```python
from build123d import *

# Parameters (mm, degrees)
SKETCH1_R           = 57.15
BOSS_EXTRUDE1_DEPTH = 2.54
SKETCH3_W           = 55.958888442
SKETCH3_H           = 22.106904705
CUT_EXTRUDE1_DEPTH  = 2.54
SKETCH4_R           = 12.7
CUT_EXTRUDE2_DEPTH  = 2.54
SKETCH5_R           = 12.7
CUT_EXTRUDE3_DEPTH  = 2.54


with BuildPart() as part:
    # Sketch1 → Boss-Extrude1 (new body)
    with BuildSketch(Plane(origin=(0, 0, 0), x_dir=(1, 0, 0), z_dir=(0, 1, 0))):
        Circle(SKETCH1_R)
    extrude(amount=BOSS_EXTRUDE1_DEPTH)

    # Sketch3 → Cut-Extrude1 (cut)
    with BuildSketch(Plane(origin=(0, 2.54, 0), x_dir=(1, 0, 0), z_dir=(0, 1, 0))):
        with Locations((-10.970545038, 0.068604303)):
            Rectangle(SKETCH3_W, SKETCH3_H)
    extrude(amount=-CUT_EXTRUDE1_DEPTH, mode=Mode.SUBTRACT)

    # Sketch4 → Cut-Extrude2 (cut)
    with BuildSketch(Plane(origin=(0, 0, 0), x_dir=(-1, 0, 0), z_dir=(0, -1, 0))):
        with Locations((50.8, 0)):
            Circle(SKETCH4_R)
    extrude(amount=-CUT_EXTRUDE2_DEPTH, mode=Mode.SUBTRACT)

    # Sketch5 → Cut-Extrude3 (cut)
    with BuildSketch(Plane.XZ):
        with Locations((50.8, 0)):
            Circle(SKETCH5_R)
    extrude(amount=-CUT_EXTRUDE3_DEPTH, mode=Mode.SUBTRACT)


solid = part.part
```
Source: CAD feature listing. Evaluate the final solid. Frame: model axes, mm. A direction names the side the tool comes from. Round coordinates to 2 decimals unless told otherwise and drop trailing zeros. Loops run counter-clockwise (first coordinate to the right, second up) from the corner with the lowest first, then second, coordinate; pieces in that order, holes last. Notation, with made-up numbers: M -9,-22 L 9,-22 A36 cw 9,15 Z; hole C 28.25,72 d9. An arc over 180 degrees is marked long. Use a Markdown table: item, result. Add a question column.
1. Pull-direction query (X, two-part tool) for faces 3 (the flat face through (-1, 2.54, 12)), 4 (the flat face through (17.009, 1, 0)), 5 (the cylindrical face through (-1.09, 1.25, 57.14)); classes: +X half, -X half, draft (parallel to the pull), parting line (faces both ways), or undercut.
2. Contact query for flat-ended pins moving along their axis: pin 1 (12 mm diameter, centred on x = 21.5, z = 9.5, fed in from -Y); pin 2 (1.5 mm diameter, centred on x = -43, y = 2, fed in from -Z); pin 3 (1.3 mm diameter, centred on y = 1, z = 7.5, fed in from +X); pin 4 (0.8 mm diameter, centred on y = 1.5, z = 2.5, fed in from -X). Output: stop coordinate, or through.
3. Cut plane A-A, the plane x = 50.8. Output: boundary loops of the cut face in (y, z), and give its area (3 significant figures).
4. Cut plane B-B, the plane y = 0.8. Output: boundary loops of the cut face in (x, z).
5. Cut plane C-C, the plane x = -23. Output: boundary loops of the cut face in (y, z).
6. Ray query, line 1 along X through (y, z) = (0.55, 0); line 2 along Z through (x, y) = (5, 1.55); line 3 along Z through (x, y) = (1, 1.95). Return the intervals inside material, ascending. Write a range as [from, to].
7. Set-up query: faces 1 (the flat face through (-1, 0, 12)), 2 (the flat face through (-38.95, 1, 8)). Return all of +Z, -Z, +X, -X, +Y, -Y with unobstructed straight access to the full face (end or side cutting, diameter ignored); none if empty.
8. Cut plane D-D, the plane z = 0. Output: boundary loops of the cut face in (x, y).
Solution:
| question | item | result |
|---|---|---|
| 1 | face 3 | draft |
| 1 | face 4 | undercut |
| 1 | face 5 | parting line |
| 2 | pin 1 | stops at y = 0 |
| 2 | pin 2 | stops at z = -38.48 |
| 2 | pin 3 | stops at x = 41.06 |
| 2 | pin 4 | stops at x = 17.01 |
| 3 | outline | M 0,-26.18 L 2.54,-26.18 L 2.54,-12.7 L 0,-12.7 Z; M 0,12.7 L 2.54,12.7 L 2.54,26.18 L 0,26.18 Z |
| 3 | area | 68.5 mm2 |
| 4 | outline | M -55.96,-11.6 A57.15 ccw 55.96,-11.6 A12.7 cw long 55.96,11.6 A57.15 ccw -55.96,11.6 A12.7 cw -38.95,4.57 L -38.95,10.98 L 17.01,10.98 L 17.01,-11.12 L -38.95,-11.12 L -38.95,-4.57 A12.7 cw Z |
| 5 | outline | M 0,-52.32 L 2.54,-52.32 L 2.54,-11.12 L 0,-11.12 Z; M 0,10.98 L 2.54,10.98 L 2.54,52.32 L 0,52.32 Z |
| 6 | line 1 | x = [17.01, 38.1] |
| 6 | line 2 | z = [-56.93, -11.12], [10.98, 56.93] |
| 6 | line 3 | z = [-57.14, -11.12], [10.98, 57.14] |
| 7 | face 1 | +Z, -Z, +X, -X, -Y |
| 7 | face 2 | +Y, -Y |
| 8 | outline | M 17.01,0 L 38.1,0 L 38.1,2.54 L 17.01,2.54 Z |
